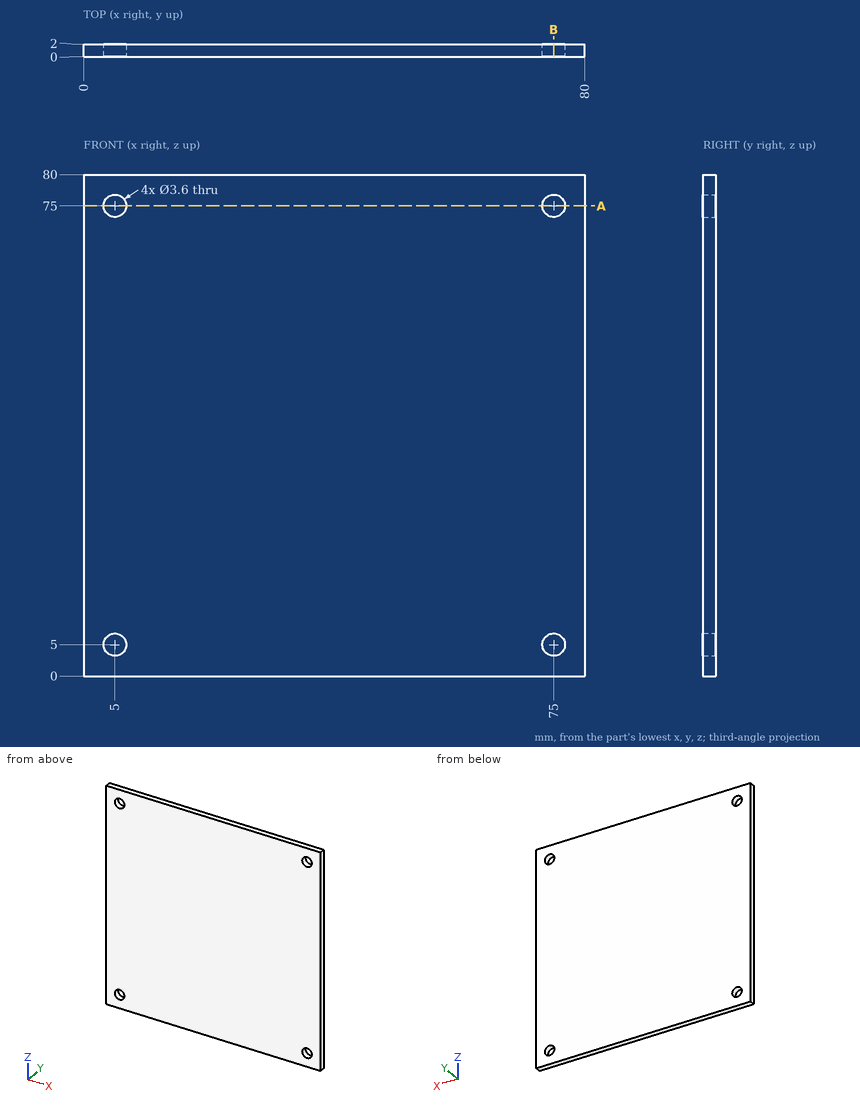
Job drawing, mm, ordinate dimensions from the low corner. One solid piece. Round coordinates to 2 decimals unless told otherwise and drop trailing zeros. Write each loop counter-clockwise with the first axis right and the second up, starting at its lowest first coordinate (ties: lowest second). Pieces come first, ordered by that corner, then holes. Notation, with made-up numbers: M -12,-17 L 47,-17 A6 ccw 47,-7 Z; hole C -13,-28.5 d2. An arc over 180 degrees is marked long. Return JSON: item names as keys, results as strings. Group by question number.
(1) Saw through at B-B on x = 75. Write the cut outline in (y, z), then the cut area to 3 significant figures.
(2) Saw through at A-A on z = 75. Write the cut outline in (x, y).
(3) Drill centre lines: probe 1 along X at (y, z) = (1.3, 5); probe 2 along Z at (x, y) = (75.5, 0.65). Where is each one in solid material? Low to high.
(4) Pin check, flat tips, straight feed: pin 1 Ø2 at (x, z) = (5, 75) entering from +Y; pin 2 Ø4.5 at (x, z) = (75, 5) entering from -Y. Stop position of each tip, or through.
Returned:
{
 "1": {"outline": "M 0,0 L 2,0 L 2,3.2 L 0,3.2 Z; M 0,6.8 L 2,6.8 L 2,73.2 L 0,73.2 Z; M 0,76.8 L 2,76.8 L 2,80 L 0,80 Z", "area": "146 mm²"},
 "2": {"outline": "M 0,0 L 3.2,0 L 3.2,2 L 0,2 Z; M 6.8,0 L 73.2,0 L 73.2,2 L 6.8,2 Z; M 76.8,0 L 80,0 L 80,2 L 76.8,2 Z"},
 "3": {"probe 1": "0 to 3.2, 6.8 to 73.2, 76.8 to 80", "probe 2": "0 to 3.27, 6.73 to 73.27, 76.73 to 80"},
 "4": {"pin 1": "through", "pin 2": "y = 0"}
}
